```python
from build123d import *

# Parameters (mm, degrees)
EXTRUDE_1_DEPTH                 = 6
CUT_EXTRUDE_1_REACH             = 24.039
SKETCH_2_R                      = 1.6
CUT_EXTRUDE_1_DIRECTION_2_DEPTH = 23.03886395


with BuildPart() as part:
    # 草图1 → 凸台-拉伸1 (new body)
    with BuildSketch(Plane(origin=(0, 0, 0), x_dir=(1, 0, 0), z_dir=(0, 1, 0))):
        Polygon((0, 0), (15, 0), (15, -4), (2.309401077, -4), (-4.035898385, -14.990381057), (-7.5, -12.990381057), align=None)
    extrude(amount=EXTRUDE_1_DEPTH)

    # 草图2 → 切除-拉伸1 (cut, up to next)
    with BuildSketch(Plane(origin=(0, 0, 0), x_dir=(-0.4999999999999975, 0, 0.86602540378444), z_dir=(-0.86602540378444, 0, -0.4999999999999975)), mode=Mode.PRIVATE) as cut_extrude_1_sk1:
        with Locations(Location((11, 3, 0), (0, 0, 180))):
            Circle(SKETCH_2_R)
    cut_extrude_1_tool1 = extrude(cut_extrude_1_sk1.sketch, amount=-CUT_EXTRUDE_1_REACH, mode=Mode.PRIVATE) & part.part
    cut_extrude_1 = cut_extrude_1_tool1.solids().sort_by_distance((-5.5, 3, 9.526279))[0]
    add(cut_extrude_1, mode=Mode.SUBTRACT)

    # 草图2 → 切除-拉伸1 direction 2 (cut)
    with BuildSketch(Plane(origin=(0, 0, 0), x_dir=(-0.4999999999999975, 0, 0.86602540378444), z_dir=(-0.86602540378444, 0, -0.4999999999999975))):
        with Locations(Location((11, 3, 0), (0, 0, 180))):
            Circle(SKETCH_2_R)
    cut_extrude_1_direction_2 = extrude(amount=CUT_EXTRUDE_1_DIRECTION_2_DEPTH, mode=Mode.SUBTRACT)

    # 镜向1: 切除-拉伸1, 切除-拉伸1 direction 2 across plane
    add(cut_extrude_1.mirror(Plane(origin=(0, 0, 0), x_dir=(0.5000000000000012, 0, 0.8660254037844378), z_dir=(-0.866025403784438, 0, 0.5000000000000012))), mode=Mode.SUBTRACT)
    add(cut_extrude_1_direction_2.mirror(Plane(origin=(0, 0, 0), x_dir=(0.5000000000000012, 0, 0.8660254037844378), z_dir=(-0.866025403784438, 0, 0.5000000000000012))), mode=Mode.SUBTRACT)


solid = part.part
```
Geometry check sheet. Reference: the model listing, model coordinates, mm. A direction names the side the tool comes from. Coordinates: 2 decimals unless noted, no trailing zeros. Order: outer loops, then holes, each group sorted by start corner. A loop starts at its lowest first (then second) coordinate and runs counter-clockwise, first axis right, second up.
Item 1: Section check B-B (z = 3.75). Enter the section's corners in (x, y).
Item 2: Scan lines: line 1 along Y through (x, z) = (11, 2.4); line 2 along Z through (x, y) = (13, 5.65); line 3 along X through (y, z) = (3, 2.3). Record each from-to range of solid material in increasing order.
Item 3: Section check D-D (y = 3). Enter the section's corners in (x, z), plus the area to 3 significant figures.
Item 4: Section check C-C (y = 0.85). Enter the section's corners in (x, z), plus the area to 3 significant figures.
Item 5: Tool access check on faces 1 (the flat face through (3, 6, 3.6)), 2 (the flat face through (9, 3, 4)). Record the directions out of +Z, -Z, +X, -X, +Y, -Y that give a thin tool (end or side, any length) a straight path to the whole face; none if there is none.
Item 6: Section check A-A (x = 11). Enter the section's corners in (y, z).
Item 7: Depth check by flat-ended pin: pin 1 (1 mm diameter, centred on y = 1, z = 7, fed in from -X); pin 2 (3 mm diameter, centred on x = 10.5, y = 3.5, fed in from +Z). Enter the tip coordinate at first touch or a pass-through.
Item 8: Mould release check, pull along Z, two halves, no side actions. Record for faces 3 (the flat face through (15, 3, 2)), 4 (the flat face through (-5.744, 2.958, 14.004)), 5 (the cylindrical face through (-4.427, 3.974, 11.612)), 6 (the flat face through (7, 3, 0)): released by +Z, released by -Z, zero draft, split by the parting line, or undercut.
Check sheet entries:
1. outline: (-2.17, 0) - (15, 0) - (15, 6) - (-2.17, 6) - close; hole circle Ø3.2 at (11, 3)
2. line 1: y = 0 to 1.4, 4.6 to 6
2. line 2: z = 0 to 4
2. line 3: x = -1.33 to 9.4, 12.6 to 15
3. outline: (-7.5, 12.99) - (-6.3, 10.91) - (-2.84, 12.91) - (-4.04, 14.99) - close; (-4.7, 8.14) - (0, 0) - (9.4, 0) - (9.4, 4) - (2.31, 4) - (-1.24, 10.14) - close; (12.6, 0) - (15, 0) - (15, 4) - (12.6, 4) - close
3. area: 85.2 mm2
4. outline: (-7.5, 12.99) - (0, 0) - (15, 0) - (15, 4) - (2.31, 4) - (-4.04, 14.99) - close
4. area: 111 mm2
5. face 1: +Z, -Z, +X, -X, +Y
5. face 2: +Z, +X, +Y, -Y
6. outline: (0, 0) - (1.4, 0) - (1.4, 4) - (0, 4) - close; (4.6, 0) - (6, 0) - (6, 4) - (4.6, 4) - close
7. pin 1: stops at x = -4.33
7. pin 2: stops at z = 4
8. face 3: zero draft
8. face 4: released by +Z
8. face 5: undercut
8. face 6: released by -Z
